Work out the finished part from the listing and answer in its coordinate system (mm). A direction names the side the tool comes from. Round coordinates to 2 decimals unless told otherwise and drop trailing zeros. Write each loop counter-clockwise with the first axis right and the second up, starting at its lowest first coordinate (ties: lowest second). Pieces come first, ordered by that corner, then holes. Notation, with made-up numbers: M 75.25,16 L 119.25,16 A25 ccw 119.25,36 Z; hole C 81.5,87 d6. An arc over 180 degrees is marked long. One line per item, written item: value. Start each with the question number.
Q1. Consider probe 1 along Y at (x, z) = (0, 5.85); probe 2 along Y at (x, z) = (0, 37.2); probe 3 along X at (y, z) = (1.5, 20.5). Determine where each line is inside the solid, lowest interval first.
Q2. Given pin 1 Ø0.7 at (x, z) = (0, 15.5) entering from +Y; pin 2 Ø8 at (y, z) = (7, 35) entering from -X; pin 3 Ø3 at (x, y) = (-1, -0.5) entering from +Z, each flat-ended and moving along its own axis, determine where each tip first touches the part or whether it passes through.
Q3. A tool of negligible diameter and unlimited length cuts with its end or side. For faces 5 (the cylindrical face through (-6, 0, 29)), 6 (the cylindrical face through (4.336, -19.524, 6.479)), 7 (the flat face through (-16.5, 0, 13)), from which of +Z, -Z, +X, -X, +Y, -Y can it reach the whole face along a straight path? Write none if from no direction.
Q4. The mould has two halves that part along X. Classify faces 1 (the flat face through (-18, 18, 0)), 2 (the cylindrical face through (-28, -21, 13)), 3 (the flat face through (0, -5, 13)), 4 (the flat face through (1.1, -11, 13)): released by +X, released by -X, zero draft, split by the parting line, or undercut.
Q5. Find section A-A (z = 16). Write down the section's boundary in (x, y).
Q6. Find section B-B (y = 0). Count the separate pieces of the cut face and the enclosed holes in it, and give its area (3 significant figures).
Q7. Find section D-D (z = 35). Write down the section's boundary in (x, y), and give its area (3 significant figures).
from build123d import *

# Parameters (mm, degrees)
SKETCH_1_R          = 35
EXTRUDE_1_DEPTH     = 27
SKETCH_2_R          = 20
CUT_EXTRUDE_1_DEPTH = 8
CUT_EXTRUDE_START   = -8
SKETCH_3_R          = 20
CUT_EXTRUDE_2_DEPTH = 8
FILLET_3_R          = 5
FILLET_4_R          = 5
SKETCH_4_R          = 6
EXTRUDE_2_DEPTH     = 20
SKETCH_5_R          = 3
CUT_EXTRUDE_3_DEPTH = 6
FILLET_5_R          = 1
FILLET_6_R          = 1
SKETCH_6_W          = 11.5
SKETCH_6_H          = 2.2
SKETCH_6_W_2        = 2.2
SKETCH_6_H_2        = 11.5
CUT_EXTRUDE_5_DEPTH = 11
SKETCH_7_R          = 2
EXTRUDE_3_DEPTH     = 4
FILLET_8_R          = 2


with BuildPart() as part:
    # 草图1 → 凸台-拉伸1 (new body)
    with BuildSketch(Plane.XY):
        Circle(SKETCH_1_R)
    extrude(amount=EXTRUDE_1_DEPTH)

    # 草图2 → 切除-拉伸1 (cut)
    with BuildSketch(Plane(origin=(0, 0, 0), x_dir=(-1, 0, 0), z_dir=(0, 0, -1))):
        Circle(SKETCH_2_R)
    extrude(amount=-CUT_EXTRUDE_1_DEPTH, mode=Mode.SUBTRACT)

    # 草图3 → 切除-拉伸2 (cut)
    with BuildSketch(Plane.XY.offset(27).offset(CUT_EXTRUDE_START)):
        with Locations(Location((0, 0, 0), (0, 0, 180))):
            Circle(SKETCH_3_R)
    extrude(amount=CUT_EXTRUDE_2_DEPTH, mode=Mode.SUBTRACT)

    # 圆角3
    fillet_3_edges = [part.edges().sort_by_distance(p)[0] for p in [
        (20, 0, 0),
    ]]
    fillet(fillet_3_edges, radius=FILLET_3_R)

    # 圆角4
    fillet_4_edges = [part.edges().sort_by_distance(p)[0] for p in [
        (20, 0, 27),
    ]]
    fillet(fillet_4_edges, radius=FILLET_4_R)

    # 草图4 → 凸台-拉伸2 (add)
    with BuildSketch(Plane.XY.offset(19)):
        Circle(SKETCH_4_R)
    extrude(amount=EXTRUDE_2_DEPTH)

    # 草图5 → 切除-拉伸3 (cut)
    with BuildSketch(Plane.XY.offset(39)):
        Circle(SKETCH_5_R)
    extrude(amount=-CUT_EXTRUDE_3_DEPTH, mode=Mode.SUBTRACT)

    # 圆角5
    fillet_5_edges = [part.edges().sort_by_distance(p)[0] for p in [
        (-35, 0, 0),
    ]]
    fillet(fillet_5_edges, radius=FILLET_5_R)

    # 圆角6
    fillet_6_edges = [part.edges().sort_by_distance(p)[0] for p in [
        (-35, 0, 27),
    ]]
    fillet(fillet_6_edges, radius=FILLET_6_R)

    # 草图6 → 切除-拉伸5 (cut)
    with BuildSketch(Plane(origin=(0, 0, 8), x_dir=(-1, 0, 0), z_dir=(0, 0, -1))):
        with Locations((10.75, 0)):
            Rectangle(SKETCH_6_W, SKETCH_6_H)
        with Locations((0, -10.75)):
            Rectangle(SKETCH_6_W_2, SKETCH_6_H_2)
        with Locations((0, 10.75)):
            Rectangle(SKETCH_6_W_2, SKETCH_6_H_2)
        with Locations((-10.75, 0)):
            Rectangle(SKETCH_6_W, SKETCH_6_H)
    extrude(amount=-CUT_EXTRUDE_5_DEPTH, mode=Mode.SUBTRACT)

    # 草图7 → 凸台-拉伸3 (add)
    with BuildSketch(Plane(origin=(0, 0, 8), x_dir=(-1, 0, 0), z_dir=(0, 0, -1))):
        Circle(SKETCH_7_R)
    extrude(amount=EXTRUDE_3_DEPTH)

    # 圆角8
    fillet_8_edges = [part.edges().sort_by_distance(p)[0] for p in [
        (2, 0, 4),
    ]]
    fillet(fillet_8_edges, radius=FILLET_8_R)


solid = part.part
The answers:
1. probe 1: -35 to -20, -1.99 to 1.99, 20 to 35
1. probe 2: -6 to -3, 3 to 6
1. probe 3: -34.97 to -19.94, -5.81 to 5.81, 19.94 to 34.97
2. pin 1: y = 35
2. pin 2: x = -5.2
2. pin 3: z = 33
3. face 5: +Z
3. face 6: -Z
3. face 7: +Z, -Z
4. face 1: zero draft
4. face 2: split by the parting line
4. face 3: undercut
4. face 4: undercut
5. outline: C 0,0 d70; hole M -16.5,-1.1 L -5,-1.1 L -5,1.1 L -16.5,1.1 Z; hole M -1.1,-16.5 L 1.1,-16.5 L 1.1,-5 L -1.1,-5 Z; hole M -1.1,5 L 1.1,5 L 1.1,16.5 L -1.1,16.5 Z; hole M 5,-1.1 L 16.5,-1.1 L 16.5,1.1 L 5,1.1 Z
6. separate pieces: 3
6. enclosed holes: 0
6. area: 1,190 mm2
7. outline: C 0,0 d12; hole C 0,0 d6
7. area: 84.8 mm2
